```python
from build123d import *

# Parameters (mm, degrees)
INTERMEDIATE_BODY_SK_W  = 13.97
INTERMEDIATE_BODY_SK_H  = 13.97
INTERMEDIATE_BODY_DEPTH = 19.685
PIN1_R                  = 2.3749
PIN_EXTRUDE1_DEPTH      = 12.0015
PIN2_R                  = 2.3749
PIN_EXTRUDE2_DEPTH      = 12.0015
FILLET1_R               = 1.27


with BuildPart() as part:
    # Intermediate_Body-Sk → Intermediate_Body (new body)
    with BuildSketch(Plane(origin=(0, 0, 0), x_dir=(1, 0, 0), z_dir=(0, 1, 0))):
        Rectangle(INTERMEDIATE_BODY_SK_W, INTERMEDIATE_BODY_SK_H)
    extrude(amount=INTERMEDIATE_BODY_DEPTH)

    # Rev-CutSk → Cut-Revolve2 (revolve, cut)
    with BuildSketch(Plane.XY, mode=Mode.PRIVATE) as cut_revolve2_sk:
        Polygon((-6.731, 19.685), (-13.081, 16.018825791), (-13.081, 3.666174209), (-6.731, 0), (-15.621, 0), (-15.621, 19.685), align=None)
    revolve(cut_revolve2_sk.sketch.rotate(Axis((0, 0, 0), (0, 1, 0)), 180), axis=Axis((0, 0, 0), (0, 1, 0)), mode=Mode.SUBTRACT)

    # Pin1 → Pin-Extrude1 (add, symmetric)
    with BuildSketch(Plane.XY):
        with Locations(Location((0, 6.6675, 0), (0, 0, 180))):
            Circle(PIN1_R)
    extrude(amount=PIN_EXTRUDE1_DEPTH, both=True)

    # Pin2 → Pin-Extrude2 (add, symmetric)
    with BuildSketch(Plane(origin=(0, 0, 0), x_dir=(0, 0, -1), z_dir=(1, 0, 0))):
        with Locations((0, 13.0175)):
            Circle(PIN2_R)
    extrude(amount=PIN_EXTRUDE2_DEPTH, both=True)

    # Fillet1
    fillet1_edges = [part.edges().sort_by_distance(p)[0] for p in [
        (6.985, 9.8425, -6.985),
        (-6.985, 9.8425, -6.985),
        (-6.985, 9.8425, 6.985),
        (6.985, 9.8425, 6.985),
    ]]
    fillet(fillet1_edges, radius=FILLET1_R)


solid = part.part
```
Work out the finished part from the listing and answer in its coordinate system (mm). A direction names the side the tool comes from. Give positions to 0.01 mm unless a question says otherwise; leave off trailing zeros. Order: outer loops, then holes, each group sorted by start corner. A loop starts at its lowest first (then second) coordinate and runs counter-clockwise, first axis right, second up. Notation, with made-up numbers: (66, -37.75) - (108, -37.75) arc R17 ccw to (108, -32.75) - close; hole circle Ø4 at (31.25, -37). An arc over 180 degrees is marked (long way). One line per item, written item: value. Start each with the question number.
1. Consider line 1 (X direction, y = 15.25, z = -1.5) (3 decimals); line 2 (Z direction, x = 7.5, y = 13). Determine where each line is inside the solid, lowest interval first.
2. Each of these flat-tipped pins is pushed along its axis until it touches: pin 1 Ø5 at (x, y) = (-6, 5) entering from +Z (3 decimals); pin 2 Ø4 at (x, y) = (7.5, 3) entering from -Z (3 decimals); pin 3 Ø8 at (y, z) = (2, -4) entering from -X (3 decimals); pin 4 Ø10 at (x, z) = (-6.5, 9) entering from +Y (3 decimals). Where does it stop, or does it pass through?
3. For a pull along Z with two mould halves and no side action, classify faces 5 (the face through (-6.623, 9.962, -6.603)), 6 (the face through (6.603, 9.962, 6.623)), 7 (the face through (-6.985, 10, 0)), 8 (the face through (-5.27, 0.24, -4.83)) as released by +Z, released by -Z, zero draft, split by the parting line, or undercut.
4. Section D-D, the plane x = -9 is taken. Write down the section's boundary in (y, z), then the cut area to 3 significant figures.
5. Section A-A, the plane y = 10 is taken. Write down the section's boundary in (x, z) (3 decimals), then the cut area to 3 significant figures.
6. Which of the six approach directions +Z, -Z, +X, -X, +Y, -Y give full straight-line access (tool end or side, diameter ignored) to faces 1 (the face through (12.002, 13, 0)), 2 (the face through (0.309, 4.313, -9.458)), 3 (the face through (-9.458, 15.372, 0.309)), 4 (the face through (9.528, 15.372, 0.309))?
Filled sheet:
1. line 1: -6.985 to 6.985
1. line 2: -2.37 to 2.37
2. pin 1: z = 6.985
2. pin 2: z = -6.985
2. pin 3: x = -6.985
2. pin 4: y = 19.685
3. face 5: released by -Z
3. face 6: released by +Z
3. face 7: zero draft
3. face 8: split by the parting line
4. outline: circle Ø4.75 at (13.02, 0)
4. area: 17.7 mm²
5. outline: (-6.985, -5.715) arc R1.27 ccw to (-5.715, -6.985) - (5.715, -6.985) arc R1.27 ccw to (6.985, -5.715) - (6.985, 5.715) arc R1.27 ccw to (5.715, 6.985) - (-5.715, 6.985) arc R1.27 ccw to (-6.985, 5.715) - close
5. area: 194 mm²
6. face 1: +Z, -Z, +X, +Y, -Y
6. face 2: -Z
6. face 3: -X
6. face 4: +X
